Drawing for the job (mm, zero at the part's lowest x, y, z). Coordinates: 2 decimals unless noted, no trailing zeros. Loops run counter-clockwise (first coordinate to the right, second up) from the corner with the lowest first, then second, coordinate; pieces in that order, holes last. Notation, with made-up numbers: (-21.75, 87.5) -> (-2.75, 87.5) arc R26 ccw to (-2.75, 108.5) -> close; hole circle Ø3 at (46, 85.25). An arc over 180 degrees is marked (long way). Write each question's results on one line, items separated by ' | '.
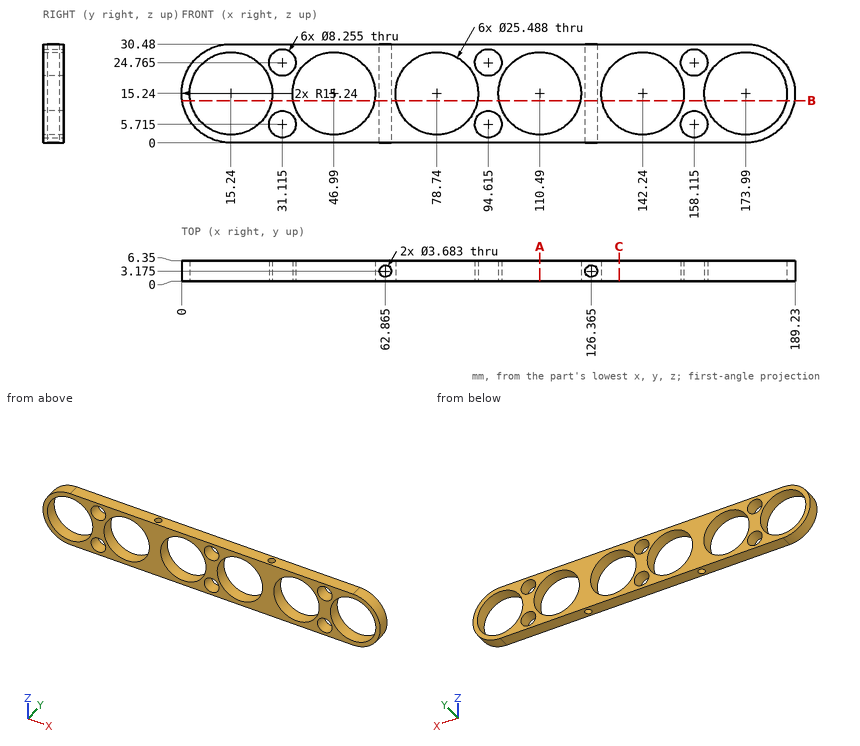
1) Drill centre lines: L1, parallel to Y at x = 63, z = 4; L2, parallel to Z at x = 169.5, y = 2; L3, parallel to Z at x = 163, y = 6.25. Where is each one in solid material? Low to high. Write a range as from..to.
Outcome:
L1: y = 0..1.34, 5.01..6.35 | L2: z = 0..3.31, 27.17..30.48 | L3: z = 0..8.79, 21.69..30.48
2) Slice it at C-C (x = 135). Write the cut outline in (y, z).
Outcome:
outline: (0, 0) -> (6.35, 0) -> (6.35, 4.75) -> (0, 4.75) -> close; (0, 25.73) -> (6.35, 25.73) -> (6.35, 30.48) -> (0, 30.48) -> close
3) Slice it at B-B (z = 13). Count the separate pieces of the cut face and the enclosed holes in it, then the cut area to 3 significant figures.
Outcome:
separate pieces: 7 | enclosed holes: 2 | area: 222 mm^2
4) Slice it at A-A (x = 110.49). Write the cut outline in (y, z).
Outcome:
outline: (0, 0) -> (6.35, 0) -> (6.35, 2.5) -> (0, 2.5) -> close; (0, 27.98) -> (6.35, 27.98) -> (6.35, 30.48) -> (0, 30.48) -> close
5) Pin check, flat tips, straight feed: pin 1 (2 mm diameter, centred on x = 62.865, y = 3.175, fed in from -Z); pin 2 (1 mm diameter, centred on y = 3.5, z = 13.5, fed in from -X). Stop position of each tip, or through.
Outcome:
pin 1: passes through | pin 2: stops at x = 0.05
